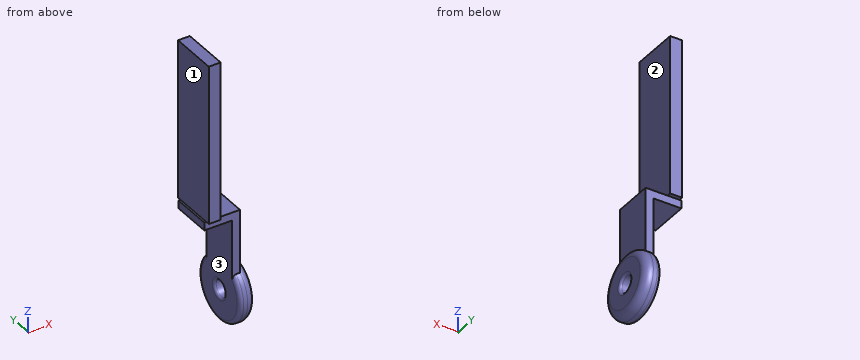
from build123d import *

# Parameters (mm, degrees)
F0_R      = 10.16
F1_DEPTH  = 2.54
F2_R      = 2.667
F3_DEPTH  = 26.02296
F4_R      = 10.16
F5_DEPTH  = 5.08
F7_R      = 2.667
F8_DEPTH  = 61.29661
F9_DEPTH  = 2.54
F10_W     = 8.89
F10_H     = 12.7
F11_DEPTH = 2.54
F13_DEPTH = 50.8
F14_R     = 2.53999
F15_R     = 1.27
F16_R     = 0.762


# Not quite as in the source:
# - a fillet or chamfer is up to 0.001 mm smaller than in the source, because OpenCascade refuses the exact size


with BuildPart() as f1:
    # F0 (on Right) → F1 (new body)
    with BuildSketch(Plane.YZ):
        Circle(F0_R)
    extrude(amount=-F1_DEPTH)

    # F2 (on face) → F3 (cut)
    with BuildSketch(Plane(origin=(-2.54, 0, 0), x_dir=(0, -1, 0), z_dir=(-1, 0, 0))):
        Circle(F2_R)
    extrude(amount=-F3_DEPTH, mode=Mode.SUBTRACT)

    # F4 (on Right) → F5 (join)
    with BuildSketch(Plane.YZ):
        Circle(F4_R)
    extrude(amount=-F5_DEPTH)

    # F7 (on face) → F8 (cut)
    with BuildSketch(Plane(origin=(-5.08, 0, 0), x_dir=(0, -1, 0), z_dir=(-1, 0, 0))):
        Circle(F7_R)
    extrude(amount=-F8_DEPTH, mode=Mode.SUBTRACT)

    # F6 (on face) → F9 (join)
    with BuildSketch(Plane(origin=(-5.08, 0, 0), x_dir=(0, -1, 0), z_dir=(-1, 0, 0))):
        with BuildLine():
            Line((-6.35, 28.251147458), (-6.35, 7.931147458))
            ThreePointArc((-6.35, 7.931147458), (0, 10.16), (6.35, 7.931147458))
            Line((6.35, 7.931147458), (6.35, 28.251147458))
            Line((6.35, 28.251147458), (-6.35, 28.251147458))
        make_face()
    extrude(amount=-F9_DEPTH)

    # F10 (on face) → F11 (join)
    with BuildSketch(Plane.XY.offset(28.251147458)):
        with Locations((-9.525, 0)):
            Rectangle(F10_W, F10_H)
    extrude(amount=-F11_DEPTH)

    # F12 (on face) → F13 (join)
    with BuildSketch(Plane.XY.offset(28.251147458)):
        Polygon((-9.5504, 7.62), (-13.335, 7.62), (-13.335, -7.62), (-9.5504, -7.62), (-9.5504, 0), align=None)
    extrude(amount=F13_DEPTH)

    # F14 (radius 2.54 in the source; OpenCascade refuses exactly that, so slightly less here)
    f14_edges = [f1.edges().sort_by_distance(p)[0] for p in [
        (0, -10.16, 0),
    ]]
    fillet(f14_edges, radius=F14_R)

    # F15
    f15_edges = [f1.edges().sort_by_distance(p)[0] for p in [
        (-5.08, -4.399409, -9.1581),
    ]]
    fillet(f15_edges, radius=F15_R)

    # F16
    f16_edges = [f1.edges().sort_by_distance(p)[0] for p in [
        (-5.08, 2.667, 0),
        (0, 2.667, 0),
    ]]
    fillet(f16_edges, radius=F16_R)


solid = f1.part
Work out the finished part from the listing and answer in its coordinate system (mm). Face numbers are marked on the shaded views. A direction names the side the tool comes from. Coordinates: 2 decimals unless noted, no trailing zeros. Loops run counter-clockwise (first coordinate to the right, second up) from the corner with the lowest first, then second, coordinate; pieces in that order, holes last. Notation, with made-up numbers: M 14.25,22.5 L 60.25,22.5 A13 cw 60.25,37.5 Z; hole C 3,-23.5 d7. An arc over 180 degrees is marked long. Answer in a Markdown table with one row per item. Add a question column.
1. A tool of negligible diameter and unlimited length cuts with its end or side. For the marked faces 1, 2 and 3, from which of +Z, -Z, +X, -X, +Y, -Y can it reach the whole face along a straight path? Write none if from no direction.
2. Consider L1, parallel to Z at x = -3, y = 0; L2, parallel to Z at x = -7, y = -1; L3, parallel to X at y = -7.5, z = 39.5 (3 decimals). Determine where each line is inside the solid, lowest interval first.
3. Find section B-B, the plane z = 44. Write down the section's boundary in (x, y) (3 decimals).
4. Flat-ended cylindrical pins translate along their axes: P1, Ø0.6, axis at x = -12, y = -7, coming from the -Z side; P2, Ø2.5, axis at x = -10.5, y = -1.5, coming from the -Z side; P3, Ø7, axis at y = 0, z = 0, coming from the -X side; P4, Ø5.5, axis at x = -7.5, y = 2, coming from the +Z side. Find the tip coordinate at first contact, or state that the pin passes through.
Reported:
| question | item | result |
|---|---|---|
| 1 | face 1 | +Z, -X, +Y, -Y |
| 1 | face 2 | +Z, +X, +Y, -Y |
| 1 | face 3 | -Z, -X, +Y, -Y |
| 2 | L1 | z = -10.16 to -2.67, 2.67 to 28.25 |
| 2 | L2 | z = 25.71 to 28.25 |
| 2 | L3 | x = -13.335 to -9.55 |
| 3 | outline | M -13.335,-7.62 L -9.55,-7.62 L -9.55,7.62 L -13.335,7.62 Z |
| 4 | P1 | stops at z = 28.25 |
| 4 | P2 | stops at z = 25.71 |
| 4 | P3 | stops at x = -5.08 |
| 4 | P4 | stops at z = 79.05 |
